Could you check a few things on this drawing? It's one solid part, dimensions in mm from its lowest x, y, z. Coordinates: 2 decimals unless noted, no trailing zeros. Loops run counter-clockwise (first coordinate to the right, second up) from the corner with the lowest first, then second, coordinate; pieces in that order, holes last. Notation, with made-up numbers: M 75.5,74 L 93.5,74 A27 cw 93.5,93 Z; hole C 82.5,62.25 d1. An arc over 180 degrees is marked long. Use one line per item in the form item = value. Start each with the question number.
(1) Imagine slicing it at C-C, the plane z = 27.75. Please give me the cut outline in (x, y).
(2) Imagine slicing it at B-B, the plane x = 13. Please give me the cut outline in (y, z).
(3) Will this pin go through, and if not, where does the flat tip stop? P1, Ø0.8, axis at x = 13.5, y = 1, coming from the -Z side.
(4) Imagine slicing it at A-A, the plane y = 0.45. Please give me the cut outline in (x, z), and give its area (3 significant figures).
(5) Please list where these lines run through material, in increasing order: L1, parallel to Z at x = 14.5, y = 0.25; L2, parallel to Z at x = 7.5, y = 1.1; L3, parallel to X at y = 0.7, z = 27.5.
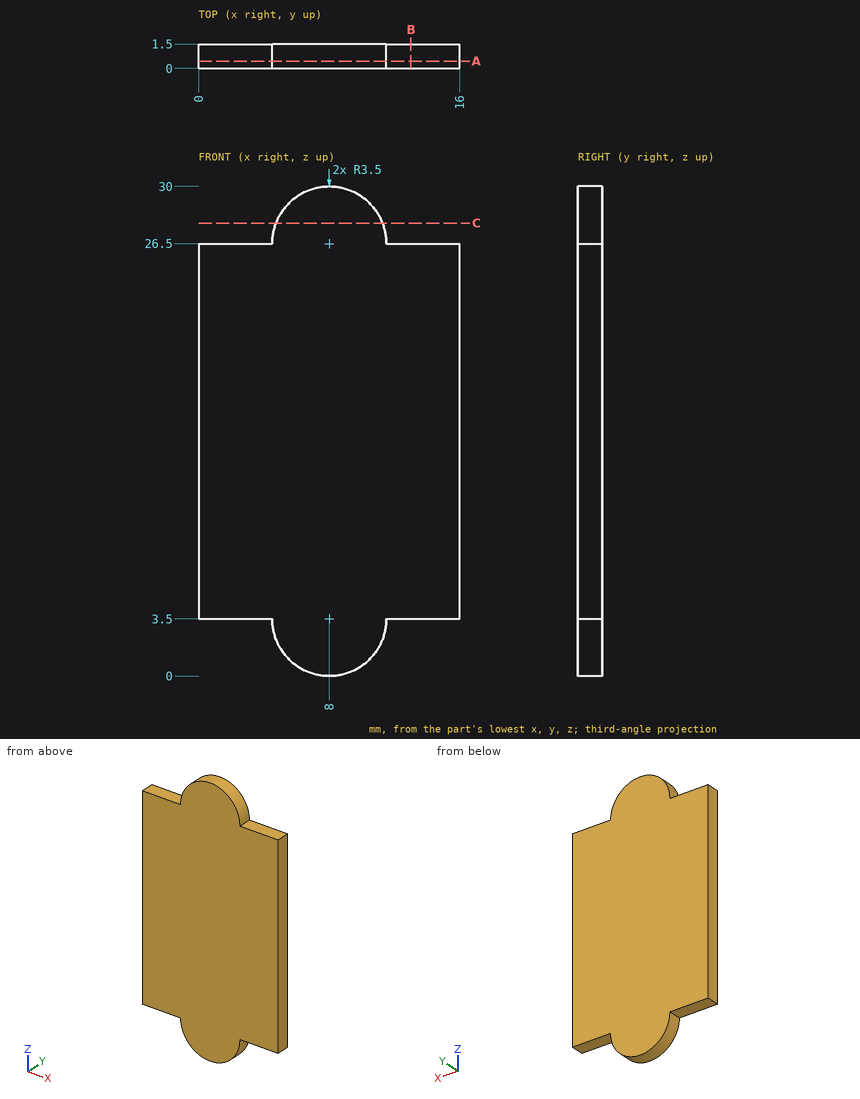
Answer:
q1.outline = M 4.73,0 L 11.27,0 L 11.27,1.5 L 4.73,1.5 Z
q2.outline = M 0,3.5 L 1.5,3.5 L 1.5,26.5 L 0,26.5 Z
q3.P1 = 3.5
q4.outline = M 0,3.5 L 4.5,3.5 A3.5 ccw 11.5,3.5 L 16,3.5 L 16,26.5 L 11.5,26.5 A3.5 ccw 4.5,26.5 L 0,26.5 Z
q4.area = 406 mm²
q5.L1 = 3.5 to 26.5
q5.L2 = 0.04 to 29.96
q5.L3 = 4.65 to 11.35
